Autodesk Inventor part; units mm, degrees
ref_plane "Pracovní rovina2" through (10, 0, 0) normal (1, 0, 0) x (0, 0, -1)
ref_plane "YZ Plane" through (0, 0, 0) normal (1, 0, 0) x (0, 1, 0)
ref_plane "XZ Plane" through (0, 0, 0) normal (0, 1, 0) x (-1, 0, 0)
ref_plane "Pracovní rovina2" through (10, 0, 0) normal (1, 0, 0) x (0, 0, -1)
sketch "Náčrt1" plane through (10, 0, 0) normal (1, 0, 0) x (0, 0, -1)
  arc A0 (-3.3166, 5) -> (-3.3166, -5) centre (0, 0) ccw
  line L0 (3.3166, 5) -> (-3.3166, 5)
  arc A1 (3.3166, -5) -> (3.3166, 5) centre (0, 0) ccw
  line L1 (-3.3166, -5) -> (3.3166, -5)
  point P0 (0, 0)
extrude "Vysunutí1" add sketch "Náčrt1" along normal blind 15
sketch "Náčrt2" plane through (25, 0, 0) normal (1, 0, 0) x (0, 0, -1)
  line L0 (-6, 5) -> (-6, -5)
  line L1 (6, 5) -> (-6, 5)
  line L2 (6, 5) -> (6, -5)
  line L3 (-6, -5) -> (6, -5)
  point P0 (0, 0)
extrude "Vysunutí2" add sketch "Náčrt2" along normal blind 9
sketch "Náčrt3" plane through (34, 0, 0) normal (1, 0, 0) x (0, 0, -1)
  arc A0 (-1.3795, -0.589) -> (-0.4321, 1.4364) centre (0, 0) ccw
  line L0 (-1.3795, -0.589) -> (-0.4321, 1.4364)
  circle A1 centre (0, 0) radius 2
  arc A2 (-0.4321, 1.4364) -> (-1.3795, -0.589) centre (0, 0) ccw
extrude "Vysunutí3" add sketch "Náčrt3" along normal blind 1
extrude "Vysunutí4" add sketch "Náčrt3" along normal blind 10 contours L0 A0
extrude "Vysunutí5" add sketch "Náčrt3" along normal blind 1.8 contours A2 L0
sketch "Náčrt4" plane through (10, 0, 0) normal (-1, 0, 0) x (0, 0, 1)
  circle A0 centre (0, 0) radius 2.5
  dimension "d12" = 5
extrude "Vysunutí6" add sketch "Náčrt4" along normal blind 0.8
fillet "Zaoblení2" radius 0.5 1 edges at (34, 0, 2)
properties part number "GA12-N20 Motor_finalV"
Input: part model. Units: mm. Frame: model coordinates. A direction names the side the tool comes from. Coordinates: 2 decimals unless noted, no trailing zeros. Loops run counter-clockwise (first coordinate to the right, second up) from the corner with the lowest first, then second, coordinate; pieces in that order, holes last.
(1) First-contact query: pin 1 Ø3 at (y, z) = (1.5, 4.5) entering from -X; pin 2 Ø4 at (y, z) = (1.5, -3.5) entering from -X; pin 3 Ø6 at (x, z) = (39, 3) entering from +Y. Flat tips, straight axial feed; report the tip coordinate or a pass-through.
(2) Section D-D on y = -4.5. Return the cut outline in (x, z).
(3) Section A-A on z = 0. Return the cut outline in (x, y), then the cut area to 3 significant figures.
(4) Set-up query: faces 1 (the face through (34.746, 1.952, 0.434)), 2 (the face through (25, 2.2, 5.8)), 3 (the face through (9.61, 2.44, -0.54)), 4 (the face through (39.843, 0.41, 0.912)), 5 (the face through (17, 0, -6)). Return all of +Z, -Z, +X, -X, +Y, -Y with unobstructed straight access to the full face (end or side cutting, diameter ignored); none if empty.
(5) Material intervals for probe 1 along X at (y, z) = (3.25, 1); probe 2 along X at (y, z) = (2.75, -5.5); probe 3 along Z at (x, y) = (37, 0.25), sorted ascending.
(6) Section C-C on x = 22. Return the cut outline in (y, z), then the cut area to 3 significant figures.
(7) Section B-B on y = 4. Return the cut outline in (x, z), then the cut area to 3 significant figures.
Data:
1. pin 1: stops at x = 10
1. pin 2: stops at x = 9.2
1. pin 3: stops at y = 1.5
2. outline: (10, -3.97) - (25, -3.97) - (25, -6) - (34, -6) - (34, 6) - (25, 6) - (25, 3.97) - (10, 3.97) - close
3. outline: (9.2, -2.5) - (10, -2.5) - (10, -5) - (34, -5) - (34, -2.5) arc R0.5 cw to (34.5, -2) - (35, -2) - (35, -1.5) - (44, -1.5) - (44, 1.5) - (35, 1.5) - (35, 2) - (34.5, 2) arc R0.5 cw to (34, 2.5) - (34, 5) - (10, 5) - (10, 2.5) - (9.2, 2.5) - close
3. area: 275 mm2
4. face 1: +X
4. face 2: +Z, -X
4. face 3: -X
4. face 4: +Z, +X, +Y
4. face 5: -Z, -X
5. probe 1: x = 10 to 34
5. probe 2: x = 25 to 34
5. probe 3: z = -1.48 to 0.99
6. outline: (-5, -3.32) arc R6 ccw to (5, -3.32) - (5, 3.32) arc R6 ccw to (-5, 3.32) - close
6. area: 104 mm2
7. outline: (10, -4.47) - (25, -4.47) - (25, -6) - (34, -6) - (34, 6) - (25, 6) - (25, 4.47) - (10, 4.47) - close
7. area: 242 mm2
